Geometry check sheet. Reference: drawing and pictorial views, mm from the part's lowest x, y, z. Round coordinates to 2 decimals unless told otherwise and drop trailing zeros. Write each loop counter-clockwise with the first axis right and the second up, starting at its lowest first coordinate (ties: lowest second). Pieces come first, ordered by that corner, then holes. Notation, with made-up numbers: M 37,-17.5 L 44,-17.5 A36 cw 44,21.5 Z; hole C 44,15.25 d10. An arc over 180 degrees is marked long. Put each result on its own line as item: value. Start each with the question number.
(1) Gauge pin test, flat ends, axial feed: pin 1 (2 mm diameter, centred on y = 7.5, z = 9.5, fed in from +X); pin 2 (6 mm diameter, centred on y = 2, z = 8.5, fed in from +X). Record the tip position at first contact, or that the pin passes through.
(2) Section check B-B on z = 10. Record the cut outline in (x, y), then the cut area to 3 significant figures.
(3) Section check A-A on y = 11. Record the cut outline in (x, z).
(4) Material ranges on probe 1 along X at (y, z) = (2.5, 13.5); probe 2 along X at (y, z) = (14.5, 9.5), recorded low to high.
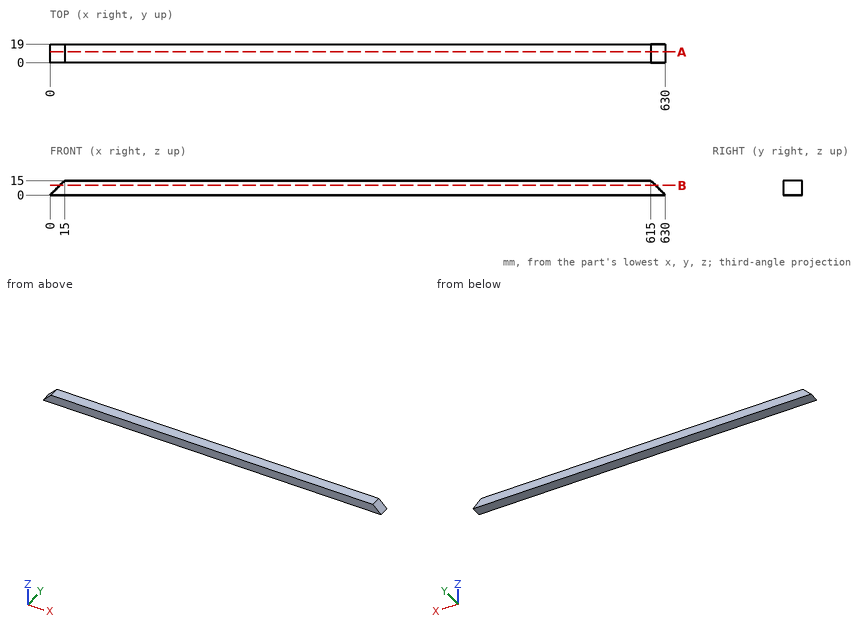
Answers follow:
1. pin 1: stops at x = 621.5
1. pin 2: stops at x = 624.5
2. outline: M 10,0 L 620,0 L 620,19 L 10,19 Z
2. area: 11,600 mm^2
3. outline: M 0,0 L 630,0 L 615,15 L 15,15 Z
4. probe 1: x = 13.5 to 616.5
4. probe 2: x = 9.5 to 620.5
